The listing builds one solid part. Answer for the finished solid, in the listing's coordinates (mm). A direction names the side the tool comes from. Coordinates: 2 decimals unless noted, no trailing zeros. Loops run counter-clockwise (first coordinate to the right, second up) from the corner with the lowest first, then second, coordinate; pieces in that order, holes last. Notation, with made-up numbers: (59.25, 1) - (86.25, 1) arc R24 ccw to (86.25, 40) - close; hole circle Ø6 at (3, 17). An arc over 180 degrees is marked (long way). Put each result on its own line as item: value.
Autodesk Inventor part; units mm, degrees
ref_plane "Work Plane1" through (0, 0, 5) normal (1, 0, 0) x (0, 0, -1)
ref_plane "YZ Plane" through (0, 0, 0) normal (1, 0, 0) x (0, 1, 0)
ref_plane "XZ Plane" through (0, 0, 0) normal (0, 1, 0) x (-1, 0, 0)
sketch "Sketch1" plane through (0, 0, 0) normal (0, 0, 1) x (1, 0, 0)
  line L0 (-22.5, 17.95) -> (22.5, 17.95)
  line L1 (22.5, 17.95) -> (22.5, -17.95)
  line L2 (22.5, -17.95) -> (-22.5, -17.95)
  line L3 (-22.5, -17.95) -> (-22.5, 17.95)
  line L4 (-29.5, 3) -> (29.5, 3)
  line L5 (29.5, 3) -> (29.5, -3)
  line L6 (29.5, -3) -> (-29.5, -3)
  line L7 (-29.5, -3) -> (-29.5, 3)
  line L8 (-22.5, -17.95) -> (22.5, 17.95) construction
  line L9 (-22.5, 17.95) -> (22.5, -17.95) construction
  line L10 (29.5, 3) -> (-29.5, -3) construction
  line L11 (-29.5, 3) -> (29.5, -3) construction
  point P0 (0, 0)
  point P1 (0, 0)
  point P2 (0, 0)
  dimension "d8" = 35.9
  dimension "d9" = 45
  dimension "d10" = 6
  dimension "d11" = 59
extrude "Extrusion1" add sketch "Sketch1" along normal blind 5
sketch "Sketch2" plane through (0, 0, 0) normal (0, 0, -1) x (-1, 0, 0)
  circle A0 centre (0, 0) radius 2.05
  circle A1 centre (-18, 13) radius 2
  line L0 (0, 0) -> (16.3137, 0) construction
  line L1 (0, 0) -> (0, -11.5343) construction
  circle A2 centre (18, 13) radius 2
  circle A3 centre (-18, -13) radius 2
  circle A4 centre (18, -13) radius 2
  dimension "d2" = 4
  dimension "d3" = 36
  dimension "d4" = 26
  dimension "d5" = 4.1
extrude "Extrusion2" cut sketch "Sketch2" against normal blind 5
sketch "Sketch3" plane through (-29.5, 3, 0) normal (0, 1, 0) x (1, 0, 0)
  line L0 (0, 0) -> (0, -5)
  line L1 (0, 0) -> (7, 0)
  line L2 (1.0635, -2) -> (4.9365, -2)
  line L3 (4.9365, -3) -> (1.0635, -3)
  arc A0 (1.0635, -3) -> (4.9365, -3) centre (3, -2.5) ccw
  arc A1 (4.9365, -2) -> (1.0635, -2) centre (3, -2.5) ccw
  point P0 (29.5, 0)
  dimension "d13" = 3
  dimension "d14" = 2.5
  dimension "d15" = 0.5
  dimension "d16" = 0.5
  dimension "d19" = 2
  dimension "d20" = 2
extrude "Extrusion3" add sketch "Sketch3" along normal blind 6 and the other way blind 11
sketch "Sketch4" plane through (-29.5, 9, 0) normal (0, 1, 0) x (1, 0, 0)
  line L0 (1.0635, -2) -> (4.9365, -2)
  arc A0 (4.9365, -2) -> (1.0635, -2) centre (3, -2.5) ccw
  line L1 (4.9365, -3) -> (1.0635, -3)
  arc A1 (1.0635, -3) -> (4.9365, -3) centre (3, -2.5) ccw
  line L2 (1.0635, -1.7) -> (4.9365, -1.7)
  arc A2 (4.9365, -1.7) -> (1.0635, -1.7) centre (3, -2.3) ccw
  line L3 (1.0635, -2) -> (1.0635, -1.7)
  line L4 (4.9365, -1.7) -> (4.9365, -2)
  line L5 (3, -2.5) -> (0.4845, -2.5) construction
  arc A3 (1.0635, -3) -> (4.9365, -3) centre (3, -2.5) ccw
  line L6 (1.0635, -3.3) -> (4.9365, -3.3)
  arc A4 (1.0635, -3.3) -> (4.9365, -3.3) centre (3, -2.7) ccw
  line L7 (1.0635, -3) -> (1.0635, -3.3)
  line L8 (4.9365, -3) -> (4.9365, -3.3)
  point P0 (29.5, 0)
  dimension "d32" = 0.2
  dimension "d33" = 0.3
extrude "Extrusion4" add sketch "Sketch4" along normal blind 2
sketch "Sketch5" plane through (-29.5, -8, 0) normal (0, -1, 0) x (1, 0, 0)
  line L0 (4.9365, 2) -> (1.0635, 2)
  arc A0 (1.0635, 2) -> (4.9365, 2) centre (3, 2.5) ccw
  line L1 (1.0635, 3) -> (4.9365, 3)
  arc A1 (4.9365, 3) -> (1.0635, 3) centre (3, 2.5) ccw
  line L2 (4.9365, 1.7) -> (1.0635, 1.7)
  arc A2 (1.0635, 1.7) -> (4.9365, 1.7) centre (3, 2.2) ccw
  line L3 (4.9365, 1.7) -> (4.9365, 2)
  line L4 (1.0635, 2) -> (1.0635, 1.7)
  line L5 (3, 2.5) -> (4.482, 2.5)
  line L6 (4.9365, 3.3) -> (1.0635, 3.3)
  arc A3 (4.9365, 3.3) -> (1.0635, 3.3) centre (3, 2.8) ccw
  line L7 (4.9365, 3.3) -> (4.9365, 3)
  line L8 (1.0635, 3) -> (1.0635, 3.3)
  point P0 (29.5, 0)
  dimension "d35" = 0.3
  dimension "d36" = 0.3
  dimension "d37" = 2
extrude "Extrusion5" add sketch "Sketch5" along normal blind 2
sketch "Sketch7" plane through (0, 0, 5) normal (0, 0, 1) x (1, 0, 0)
  circle A0 centre (18, -13) radius 2
  circle A1 centre (-18, 13) radius 2
  circle A2 centre (18, 13) radius 2
  circle A3 centre (-18, -13) radius 2
  circle A4 centre (0, 0) radius 2.05
  line L0 (-22.5, -3) -> (-22.5, -17.95)
  line L1 (-22.5, -17.95) -> (22.5, -17.95)
  line L2 (22.5, -17.95) -> (22.5, -3)
  line L3 (22.5, -3) -> (29.5, -3)
  line L4 (29.5, -3) -> (29.5, 3)
  line L5 (29.5, 3) -> (22.5, 3)
  line L6 (22.5, 3) -> (22.5, 17.95)
  line L7 (22.5, 17.95) -> (-22.5, 17.95)
  line L8 (-22.5, 17.95) -> (-22.5, 3)
  line L9 (-22.5, 3) -> (-29.5, 3)
  line L10 (-29.5, 3) -> (-29.5, -3)
  line L11 (-29.5, -3) -> (-22.5, -3)
ref_plane "Work Plane1" through (0, 0, 5) normal (1, 0, 0) x (0, 0, -1)
mirror "Mirror1" about plane through (0, 0, 5) normal (1, 0, 0) of "Extrusion3", "Extrusion4", "Extrusion5"
chamfer "Chamfer1" distance 1 angle 45 2 edges at (-26.5, 11, 0.2727) (-26.5, 11, 4.7273)
chamfer "Chamfer2" distance 1 angle 45 6 edges at (-26.5, -10, 0.2) (-26.5, -10, 4.8) (26.5, 11, 0.2727) (26.5, 11, 4.7273) (26.5, -10, 0.2) (26.5, -10, 4.8)
properties part number "mover01"
1) The part is cut by section A-A (x = -18). Give the vertices of the cut face in (y, z).
Found:
outline: (-17.95, 0) - (-15, 0) - (-15, 5) - (-17.95, 5) - close; (-11, 0) - (11, 0) - (11, 5) - (-11, 5) - close; (15, 0) - (17.95, 0) - (17.95, 5) - (15, 5) - close
2) For a pull along Z with two mould halves and no side action, classify faces 6 (the face through (27, 7, 3)), 7 (the face through (22.5, -10, 2)), 8 (the face through (26.474, 10.715, 0.988)), 9 (the face through (26.526, 10.715, 4.012)) as pulls with the +Z half, pulls with the -Z half, needs draft (parallel to the pull), parting line crosses it, or undercut.
Found:
face 6: undercut
face 7: needs draft
face 8: pulls with the -Z half
face 9: pulls with the +Z half
3) The part is cut by section D-D (y = 13). Give the vertices of the cut face in (x, z), and give its area (3 significant figures).
Found:
outline: (-22.5, 0) - (-20, 0) - (-20, 5) - (-22.5, 5) - close; (-16, 0) - (16, 0) - (16, 5) - (-16, 5) - close; (20, 0) - (22.5, 0) - (22.5, 5) - (20, 5) - close
area: 185 mm^2
4) Each of these flat-tipped pins is pushed along its axis until it touches: pin 1 (4.5 mm diameter, centred on x = -26.5, y = 8.5, fed in from -Z); pin 2 (2.5 mm diameter, centred on x = -24.5, z = 3.5, fed in from -Y); pin 3 (1.9 mm diameter, centred on x = 27.5, y = -5.5, fed in from +Z). Where does it stop, or does it pass through?
Found:
pin 1: stops at z = 0.27
pin 2: stops at y = -10
pin 3: stops at z = 4.5
5) For faces 1 (the face through (-26, -3, 2.5)), 2 (the face through (-26.5, -8.5, 4.8)), 3 (the face through (-26.536, 9.493, 0.273)), 4 (the face through (-22.5, -11, 2)), 5 (the face through (26.5, 6, 0.5)), determine the directions among +Z, -Z, +X, -X, +Y, -Y from which every point of the face is accessible in a straight line to the end or side of a thin tool.
Found:
face 1: none
face 2: +Z, -Y
face 3: -Z, +Y
face 4: +Z, -Z, -Y
face 5: -Z
6) The part is cut by section B-B (y = 5). Give the vertices of the cut face in (x, z).
Found:
outline: (-28.44, 2) arc R2 ccw to (-24.56, 2) - close; (-28.44, 3) - (-24.56, 3) arc R2 ccw to start; (-22.5, 0) - (22.5, 0) - (22.5, 5) - (-22.5, 5) - close; (24.56, 2) arc R2 ccw to (28.44, 2) - close; (24.56, 3) - (28.44, 3) arc R2 ccw to start
7) The part is cut by section C-C (x = 0). Give the vertices of the cut face in (y, z), and give its area (3 significant figures).
Found:
outline: (-17.95, 0) - (-2.05, 0) - (-2.05, 5) - (-17.95, 5) - close; (2.05, 0) - (17.95, 0) - (17.95, 5) - (2.05, 5) - close
area: 159 mm^2
8) Straight lines are drawn through the part: L1, parallel to Y at x = 18, z = 1.9; L2, parallel to Y at x = -17.5, z = 1.4; L3, parallel to X at y = 5.5, z = 3.85. For each, find the intervals that lie inside material, in ascending order. Write a range as [from, to].
Found:
L1: y = [-17.95, -15], [-11, 11], [15, 17.95]
L2: y = [-17.95, -14.94], [-11.06, 11.06], [14.94, 17.95]
L3: x = [-27.98, -25.02], [-22.5, 22.5], [25.02, 27.98]
